Work out the finished part from the listing and answer in its coordinate system (mm). A direction names the side the tool comes from. Coordinates: 2 decimals unless noted, no trailing zeros. Loops run counter-clockwise (first coordinate to the right, second up) from the corner with the lowest first, then second, coordinate; pieces in that order, holes last. Notation, with made-up numbers: (-17.5, 21.5) -> (-8.5, 21.5) arc R17 cw to (-8.5, 51.5) -> close; hole circle Ø1 at (21, 32). An arc over 180 degrees is marked (long way). Use a Markdown table: item, result. Add a question column.
```python
from build123d import *

# Parameters (mm, degrees)
SKETCH1_R           = 12.5
SKETCH1_R_2         = 2.55
BOSS_EXTRUDE1_DEPTH = 3


with BuildPart() as part:
    # Sketch1 → Boss-Extrude1 (new body)
    with BuildSketch(Plane(origin=(0, 0, 0), x_dir=(1, 0, 0), z_dir=(0, 1, 0))):
        with BuildLine():
            Line((17.75, -43.75), (-17.75, -43.75))
            ThreePointArc((-17.75, -43.75), (-19.164213562, -43.164213562), (-19.75, -41.75))
            Line((-19.75, -41.75), (-19.75, 19.25))
            ThreePointArc((-19.75, 19.25), (-19.164213562, 20.664213562), (-17.75, 21.25))
            Line((-17.75, 21.25), (17.75, 21.25))
            ThreePointArc((17.75, 21.25), (19.164213562, 20.664213562), (19.75, 19.25))
            Line((19.75, 19.25), (19.75, -41.75))
            ThreePointArc((19.75, -41.75), (19.164213562, -43.164213562), (17.75, -43.75))
        make_face()
        with Locations(Location((0, 0, 0), (0, 0, 270))):
            Circle(SKETCH1_R, mode=Mode.SUBTRACT)
        with Locations(Location((10, -38.5, 0), (0, 0, 270))):
            Circle(SKETCH1_R_2, mode=Mode.SUBTRACT)
        with Locations(Location((-10, -38.5, 0), (0, 0, 270))):
            Circle(SKETCH1_R_2, mode=Mode.SUBTRACT)
        with BuildLine():
            Line((11.903984489, 14.096015511), (14.403984489, 16.596015511))
            ThreePointArc((14.403984489, 16.596015511), (16.596015511, 16.596015511), (16.596015511, 14.403984489))
            Line((16.596015511, 14.403984489), (14.096015511, 11.903984489))
            ThreePointArc((14.096015511, 11.903984489), (11.903984489, 11.903984489), (11.903984489, 14.096015511))
        make_face(mode=Mode.SUBTRACT)
        with BuildLine():
            Line((-11.903984489, 14.096015511), (-14.403984489, 16.596015511))
            ThreePointArc((-14.403984489, 16.596015511), (-16.596015511, 16.596015511), (-16.596015511, 14.403984489))
            Line((-16.596015511, 14.403984489), (-14.096015511, 11.903984489))
            ThreePointArc((-14.096015511, 11.903984489), (-11.903984489, 11.903984489), (-11.903984489, 14.096015511))
        make_face(mode=Mode.SUBTRACT)
        with BuildLine():
            Line((-11.903984489, -14.096015511), (-14.403984489, -16.596015511))
            ThreePointArc((-14.403984489, -16.596015511), (-16.596015511, -16.596015511), (-16.596015511, -14.403984489))
            Line((-16.596015511, -14.403984489), (-14.096015511, -11.903984489))
            ThreePointArc((-14.096015511, -11.903984489), (-11.903984489, -11.903984489), (-11.903984489, -14.096015511))
        make_face(mode=Mode.SUBTRACT)
        with BuildLine():
            Line((11.903984489, -14.096015511), (14.403984489, -16.596015511))
            ThreePointArc((14.403984489, -16.596015511), (16.596015511, -16.596015511), (16.596015511, -14.403984489))
            Line((16.596015511, -14.403984489), (14.096015511, -11.903984489))
            ThreePointArc((14.096015511, -11.903984489), (11.903984489, -11.903984489), (11.903984489, -14.096015511))
        make_face(mode=Mode.SUBTRACT)
    extrude(amount=BOSS_EXTRUDE1_DEPTH)


solid = part.part
```
Item 1: For a pull along Z with two mould halves and no side action, classify faces 3 (the face through (16.57, 1.48, -16.62)), 4 (the face through (19.75, 1, 11)), 5 (the face through (-19.15, 1.48, 43.18)) as +Z half, -Z half, draft (parallel to the pull), parting line (faces both ways), or undercut.
Item 2: Section A-A (x = 0) is taken. Determine the outline of the cut face in (y, z).
Item 3: Section C-C (z = 38.5) is taken. Determine the outline of the cut face in (x, y), then the cut area to 3 significant figures.
Item 4: For faces 1 (the face through (-19.75, 1, 12)), 2 (the face through (13.14, 1.48, 15.33)), determine the directions among +Z, -Z, +X, -X, +Y, -Y from which every point of the face is accessible in a straight line to the end or side of a thin tool.
Item 5: Section B-B (y = 1.9) is taken. Determine the outline of the cut face in (x, z).
Item 6: Section D-D (z = 0) is taken. Determine the outline of the cut face in (x, y).
Item 7: Find the intervals of material crossed by probe 1 along X at (y, z) = (0.7, 38.5); probe 2 along X at (y, z) = (0.8, 0); probe 3 along Z at (x, y) = (-9.5, 2.7), in increasing order.
Output:
| question | item | result |
|---|---|---|
| 1 | face 3 | undercut |
| 1 | face 4 | draft |
| 1 | face 5 | +Z half |
| 2 | outline | (0, -21.25) -> (3, -21.25) -> (3, -12.5) -> (0, -12.5) -> close; (0, 12.5) -> (3, 12.5) -> (3, 43.75) -> (0, 43.75) -> close |
| 3 | outline | (-19.75, 0) -> (-12.55, 0) -> (-12.55, 3) -> (-19.75, 3) -> close; (-7.45, 0) -> (7.45, 0) -> (7.45, 3) -> (-7.45, 3) -> close; (12.55, 0) -> (19.75, 0) -> (19.75, 3) -> (12.55, 3) -> close |
| 3 | area | 87.9 mm2 |
| 4 | face 1 | +Z, -Z, -X, +Y, -Y |
| 4 | face 2 | +Y, -Y |
| 5 | outline | (-19.75, -19.25) arc R2 ccw to (-17.75, -21.25) -> (17.75, -21.25) arc R2 ccw to (19.75, -19.25) -> (19.75, 41.75) arc R2 ccw to (17.75, 43.75) -> (-17.75, 43.75) arc R2 ccw to (-19.75, 41.75) -> close; hole (-16.6, -14.4) arc R1.55 ccw to (-14.4, -16.6) -> (-11.9, -14.1) arc R1.55 ccw to (-14.1, -11.9) -> close; hole (-16.6, 14.4) -> (-14.1, 11.9) arc R1.55 ccw to (-11.9, 14.1) -> (-14.4, 16.6) arc R1.55 ccw to start; hole circle Ø5.1 at (-10, 38.5); hole circle Ø25 at (0, 0); hole circle Ø5.1 at (10, 38.5); hole (11.9, -14.1) -> (14.4, -16.6) arc R1.55 ccw to (16.6, -14.4) -> (14.1, -11.9) arc R1.55 ccw to start; hole (11.9, 14.1) arc R1.55 ccw to (14.1, 11.9) -> (16.6, 14.4) arc R1.55 ccw to (14.4, 16.6) -> close |
| 6 | outline | (-19.75, 0) -> (-12.5, 0) -> (-12.5, 3) -> (-19.75, 3) -> close; (12.5, 0) -> (19.75, 0) -> (19.75, 3) -> (12.5, 3) -> close |
| 7 | probe 1 | x = -19.75 to -12.55, -7.45 to 7.45, 12.55 to 19.75 |
| 7 | probe 2 | x = -19.75 to -12.5, 12.5 to 19.75 |
| 7 | probe 3 | z = -21.25 to -8.12, 8.12 to 36, 41 to 43.75 |
